Autodesk Inventor part; units mm, degrees
ref_plane "YZ Plane" through (0, 0, 0) normal (1, 0, 0) x (0, 1, 0)
ref_plane "XZ Plane" through (0, 0, 0) normal (0, 1, 0) x (-1, 0, 0)
ref_plane "XY Plane" through (0, 0, 0) normal (0, 0, 1) x (1, 0, 0)
sketch "Sketch1" plane through (0, 0, 0) normal (0, 0, 1) x (1, 0, 0)
  arc A0 (-118.3794, 10.5655) -> (-118.3794, -10.5655) centre (0, 0) ccw
  line L0 (0, 0) -> (-118.85, 0) construction
  line L1 (0, 0) -> (-118.3794, -10.5655) construction
  line L2 (-118.3794, -10.5655) -> (-118.3794, 0) construction
  line L3 (-128.85, 11.5) -> (-118.3794, 10.5655)
  line L4 (-118.3794, 0) -> (-118.3794, 10.5655) construction
  arc A1 (-128.85, 11.5) -> (-128.85, -11.5) centre (0, 0) ccw construction
  line L5 (-118.3794, 10.5655) -> (0, 0) construction
  line L6 (-118.3794, -10.5655) -> (-128.85, -11.5)
  arc A2 (-118.3794, -10.5655) -> (-118.3794, 10.5655) centre (0, 0) ccw construction
  arc A3 (-128.85, -11.5) -> (-128.85, 11.5) centre (0, 0) ccw construction
  line L7 (-128.85, 11.5) -> (-128.85, -11.5)
  dimension "d0" = 237.7
  dimension "d33" = 23
  dimension "d34" = 128.85
  dimension "d37" = 10
extrude "Extrusion1" add sketch "Sketch1" along normal mid plane 25
chamfer "Chamfer1" distance 3 angle 45 1 edges at (-118.85, 0, 12.5)
sketch "Sketch4" plane through (0, 0, 0) normal (0, 0, 1) x (1, 0, 0)
  line L0 (0, 0) -> (-126.7631, 7.7532) construction
  line L1 (0, 0) -> (-127, 0) construction
  line L2 (0, 0) -> (-126.7631, -7.7532) construction
  arc A0 (-128.85, 11.5) -> (-128.85, -11.5) centre (0, 0) ccw
  arc A1 (-121.3676, 10.8322) -> (-121.3676, -10.8322) centre (0, 0) ccw
  line L3 (-121.3676, 10.8322) -> (-128.85, 11.5)
  line L4 (-128.85, -11.5) -> (-121.3676, -10.8322)
  circle A2 centre (0, 0) radius 127 construction
  line L5 (-128.85, 11.5) -> (-128.85, -11.5)
  dimension "d25" = 3.5
  dimension "d26" = 3.5
sketch "Sketch7" plane through (0, 0, 12.5) normal (0, 0, 1) x (1, 0, 0)
  arc A0 (-121.3676, 10.8322) -> (-121.3676, -10.8322) centre (0, 0) ccw
  line L0 (-121.3676, 10.8322) -> (-128.85, 11.5)
  line L1 (-128.85, 11.5) -> (-128.85, -11.5)
  line L2 (-128.85, -11.5) -> (-121.3676, -10.8322)
  arc A1 (-123.5091, 11.0233) -> (-123.5091, -11.0233) centre (0, 0) ccw
  arc A2 (-123.5091, -11.0233) -> (-123.5091, 11.0233) centre (0, 0) ccw construction
  line L3 (-128.85, 11.5) -> (-123.5091, 11.0233)
  line L4 (-128.85, -11.5) -> (-123.5091, -11.0233)
  line L5 (-128.85, 11.4972) -> (-128.85, -11.5)
  dimension "d44" = 248
extrude "Extrusion8" add sketch "Sketch7" along normal blind 15 contours A1 L2 L1 L0
sketch "Sketch8" plane through (-128.85, -11.5, -12.5) normal (-1, 0, 0) x (0, 0, 1)
  line L0 (0, 0) -> (0, 23)
  line L1 (40, 23) -> (40, 0)
  line L2 (0, 23) -> (40, 23)
  line L3 (40, 23) -> (40, 20.1)
  line L4 (40, 20.1) -> (0, 20.1)
  line L5 (0, 20.1) -> (0, 23)
  line L6 (0, 0) -> (40, 0)
  line L7 (40, 0) -> (40, 2.9)
  line L8 (40, 2.9) -> (0, 2.9)
  line L9 (0, 2.9) -> (0, 0)
  dimension "d48" = 2.9
  dimension "d49" = 2.9
extrude "Extrusion7" add sketch "Sketch8" along normal blind 10 contours L0 L8 L1 L6 | L0 L2 L1 L4
fillet "Fillet3" radius 0.5 2 edges at (-128.85, 8.6, 7.5) (-128.85, -8.6, 7.5)
fillet "Fillet4" radius 2 5 edges at (-138.85, 10.05, 27.5) (-138.85, -10.05, 27.5) (-138.85, 10.05, -12.5) (-138.85, -10.05, -12.5) (-124, 0, 27.5)
equation "\"d26\" = d25"
equation "\"d44\" = diametro_max_soporte"
equation "\"d49\" = d48"
equation "\"angulo_alabe\" = 130deg"
equation "\"diametro_tubo\" = 232"
equation "\"desfase_a_pin_superior\" = 12"
equation "\"desfase_b_pin_inferior\" = 8"
equation "\"desfase_b_pin_superior\" = 0"
equation "\"diametro_max_soporte\" = 248"
properties part number "accesorios separador 1"
Part model, mm, in its own coordinate system. A direction names the side the tool comes from. Round coordinates to 2 decimals unless told otherwise and drop trailing zeros. Loops run counter-clockwise (first coordinate to the right, second up) from the corner with the lowest first, then second, coordinate; pieces in that order, holes last. Notation, with made-up numbers: (30, -5) -> (67, -5) arc R22 ccw to (67, 9) -> close; hole circle Ø7 at (15.5, -8.5). An arc over 180 degrees is marked (long way). Use CSV: the item, a comma, the result in double quotes. Start each with the question number.
1) Which spindle directions (+Z, -Z, +X, -X, +Y, -Y) get a long thin tool onto all of the face, cutting with end or side? Do faces 4 (the cylindrical face through (-124, 0, 19)), 5 (the flat face through (-128.85, 0, 7)), 6 (the flat face through (-138.85, 10, 7)). Say none if no direction does.
2) Cut at C-C, the plane z = 1.5. Write the cut outline in (x, y), plus the area to 3 significant figures.
3) Wall check: L1, parallel to Y at x = -133.5, z = 6; L2, parallel to Z at x = -122, y = 7; L3, parallel to X at y = 1.25, z = 4.5. Give the ranges that are in metal, low to high. Write a range as [from, to].
4) Pull direction Y, two halves, no side cores. Call faces 1 (the flat face through (-134, 11.5, 7)), 2 (the cylindrical face through (-138.25, -10.03, -11.93)), 3 (the cylindrical face through (-118.85, -0.15, -1.65)): +Y half, -Y half, draft (parallel to the pull), parting line (faces both ways), or undercut.
5) Cut at D-D, the plane x = -126.5. Write the cut outline in (y, z), plus the area to 3 significant figures.
6) Cut at B-B, the plane z = 16. Write the cut outline in (x, y), plus the area to 3 significant figures.
7) Cut at A-A, the plane x = -134. Write the cut outline in (y, z).
8) Drop flat-ended pins along their axis: P1, Ø10, axis at x = -121, z = 1, coming from the -Y side; P2, Ø1, axis at y = -2, z = -2.5, coming from the -X side; P3, Ø0.8, axis at x = -123, y = -3.5, coming from the +Z side. Give the stop position or say it passes through.
Determined:
1,face 4,"+Z, +X"
1,face 5,"+Z, -Z, -X"
1,face 6,"+Z, -Z, -X, +Y, -Y"
2,outline,"(-138.85, -11.5) -> (-128.85, -11.5) -> (-118.38, -10.57) arc R118.85 cw to (-118.38, 10.57) -> (-128.85, 11.5) -> (-138.85, 11.5) -> (-138.85, 8.6) -> (-129.35, 8.6) arc R0.5 cw to (-128.85, 8.1) -> (-128.85, -8.1) arc R0.5 cw to (-129.35, -8.6) -> (-138.85, -8.6) -> close"
2,area,"283 mm2"
3,L1,"y = [-11.5, -8.6], [8.6, 11.5]"
3,L2,"z = [-12.5, 12.5]"
3,L3,"x = [-128.85, -118.84]"
4,face 1,"+Y half"
4,face 2,"draft"
4,face 3,"undercut"
5,outline,"(-11.29, -12.5) -> (11.29, -12.5) -> (11.29, 27.5) -> (-11.29, 27.5) -> close"
5,area,"903 mm2"
6,outline,"(-138.85, -11.5) -> (-128.85, -11.5) -> (-123.51, -11.02) arc R124 cw to (-123.51, 11.02) -> (-128.85, 11.5) -> (-138.85, 11.5) -> (-138.85, 8.6) -> (-129.35, 8.6) arc R0.5 cw to (-128.85, 8.1) -> (-128.85, -8.1) arc R0.5 cw to (-129.35, -8.6) -> (-138.85, -8.6) -> close"
6,area,"171 mm2"
7,outline,"(-11.5, -12.5) -> (-8.6, -12.5) -> (-8.6, 27.5) -> (-11.5, 27.5) -> close; (8.6, -12.5) -> (11.5, -12.5) -> (11.5, 27.5) -> (8.6, 27.5) -> close"
8,P1,"stops at y = -11.25"
8,P2,"stops at x = -128.85"
8,P3,"stops at z = 12.5"
